Autodesk Inventor part; units mm, degrees
ref_plane "YZ Plane" through (0, 0, 0) normal (1, 0, 0) x (0, 1, 0)
ref_plane "XZ Plane" through (0, 0, 0) normal (0, 1, 0) x (-1, 0, 0)
ref_plane "XY Plane" through (0, 0, 0) normal (0, 0, 1) x (1, 0, 0)
sketch "Sketch1" plane through (0, 0, 0) normal (0, 0, 1) x (1, 0, 0)
  circle A0 centre (0, 0) radius 11.5
  circle A1 centre (0, 0) radius 3.25
  circle A2 centre (8.5, 0) radius 0.75
  circle A3 centre (-8.5, 0) radius 0.75
  dimension "d0" = 23
  dimension "d1" = 6.5
  dimension "d2" = 1.5
  dimension "d3" = 8.5
  dimension "d6" = 360
extrude "Extrusion1" add sketch "Sketch1" along normal blind 5
sketch "Sketch3" plane through (0, 0, 5) normal (0, 0, 1) x (1, 0, 0)
  circle A0 centre (15, 0) radius 1
  circle A1 centre (15, 0) radius 3.5
  circle A2 centre (0, 0) radius 11.5
  line L0 (6.1333, 9.7279) -> (16.8667, 2.9607)
  line L1 (16.8667, -2.9607) -> (6.1333, -9.7279)
  circle A3 centre (0, 0) radius 11.5
  arc A4 (6.1333, -9.7279) -> (6.1333, 9.7279) centre (0, 0) ccw
  circle A5 centre (-15, 0) radius 1
  circle A6 centre (-15, 0) radius 3.5
  line L2 (-6.1333, -9.7279) -> (-16.8667, -2.9607)
  line L3 (-16.8667, 2.9607) -> (-6.1333, 9.7279)
  arc A7 (-6.1333, 9.7279) -> (-6.1333, -9.7279) centre (0, 0) ccw
  dimension "d17" = 2
  dimension "d18" = 15
  dimension "d21" = 360
extrude "Extrusion3" add sketch "Sketch3" against normal blind 5 contours A1 | A1 A2 L0 | L1 A2 A1 | A2 A6 L3 | L2 A6 A2 | A6
properties part number "AC07" material "ABS Plastic"
Work out the finished part from the listing and answer in its coordinate system (mm). Coordinates: 2 decimals unless noted, no trailing zeros. Write each loop counter-clockwise with the first axis right and the second up, starting at its lowest first coordinate (ties: lowest second). Pieces come first, ordered by that corner, then holes.
1. The part is cut by section D-D, the plane x = -15. Write down the section's boundary in (y, z).
Results list:
outline: (-4.14, 0) - (-1, 0) - (-1, 5) - (-4.14, 5) - close; (1, 0) - (4.14, 0) - (4.14, 5) - (1, 5) - close
2. The part is cut by section B-B, the plane x = 0. Write down the section's boundary in (y, z), and give its area (3 significant figures).
Results list:
outline: (-11.5, 0) - (-3.25, 0) - (-3.25, 5) - (-11.5, 5) - close; (3.25, 0) - (11.5, 0) - (11.5, 5) - (3.25, 5) - close
area: 82.5 mm2
3. A flat-ended cylindrical pin translates along its axis: pin 1 (1 mm diameter, centred on x = 14.5, y = 7, fed in from -Z). Find the tip coordinate at first contact, or state that the pin passes through.
Results list:
pin 1: passes through
4. The part is cut by section A-A, the plane y = 0. Write down the section's boundary in (x, z), and give its area (4 significant figures).
Results list:
outline: (-18.5, 0) - (-16, 0) - (-16, 5) - (-18.5, 5) - close; (-14, 0) - (-9.25, 0) - (-9.25, 5) - (-14, 5) - close; (-7.75, 0) - (-3.25, 0) - (-3.25, 5) - (-7.75, 5) - close; (3.25, 0) - (7.75, 0) - (7.75, 5) - (3.25, 5) - close; (9.25, 0) - (14, 0) - (14, 5) - (9.25, 5) - close; (16, 0) - (18.5, 0) - (18.5, 5) - (16, 5) - close
area: 117.5 mm2
5. Consider line 1 along Y through (x, z) = (0, 3.45); line 2 along Y through (x, z) = (8.5, 3.85); line 3 along X through (y, z) = (4.25, 3.2). Determine where each line is inside the solid, lowest interval first.
Results list:
line 1: y = -11.5 to -3.25, 3.25 to 11.5
line 2: y = -8.24 to -0.75, 0.75 to 8.24
line 3: x = -14.82 to 14.82
6. For a pull along X with two mould halves and no side action, classify faces 1 (the cylindrical face through (-14, 0, 3)), 2 (the cylindrical face through (18.5, 0, 2.5)), 3 (the cylindrical face through (7.75, -0.03, 2.46)), 4 (the cylindrical face through (-0.1, 11.5, 2.5)) as +X half, -X half, draft (parallel to the pull), parting line (faces both ways), or undercut.
Results list:
face 1: undercut
face 2: +X half
face 3: undercut
face 4: parting line
7. The part is cut by section C-C, the plane z = 0.6. Write down the section's boundary in (x, y).
Results list:
outline: (-16.87, -2.96) - (-6.13, -9.73) arc R11.5 ccw to (6.13, -9.73) - (16.87, -2.96) arc R3.5 ccw to (16.87, 2.96) - (6.13, 9.73) arc R11.5 ccw to (-6.13, 9.73) - (-16.87, 2.96) arc R3.5 ccw to start; hole circle Ø2 at (-15, 0); hole circle Ø1.5 at (-8.5, 0); hole circle Ø6.5 at (0, 0); hole circle Ø1.5 at (8.5, 0); hole circle Ø2 at (15, 0)
